Geometry: final body of the model. Coordinates: model frame, mm. Give positions to 0.01 mm unless a question says otherwise; leave off trailing zeros. Answer in a Markdown table with one row per item. Add a question column.
Autodesk Inventor part; units mm, degrees
ref_plane "C1_XY" through (0, 0, 0) normal (0, 0, 1) x (1, 0, 0)
ref_plane "C1_YZ" through (0, 0, 0) normal (1, 0, 0) x (0, 1, 0)
ref_plane "C1_ZX" through (0, 0, 0) normal (0, 1, 0) x (0, 0, 1)
sketch "Sketch_1" plane through (0, 0, 0) normal (0, 0, 1) x (1, 0, 0)
  line L0 (-15, 4) -> (-13, 4)
  line L1 (-13, 4) -> (-13, 8.25)
  line L2 (-13, 8.25) -> (-9.6642, 8.25)
  line L3 (-9.6642, 8.25) -> (-6, 4.5858)
  line L4 (-6, 4.5858) -> (-6, 0.5196)
  line L5 (-6, 0.5196) -> (-5.7, 0)
  line L6 (-5.7, 0) -> (-6, -0.5196)
  line L7 (-6, -0.5196) -> (-6, -4.5858)
  line L8 (-6, -4.5858) -> (-9.6642, -8.25)
  line L9 (-9.6642, -8.25) -> (-13, -8.25)
  line L10 (-13, -8.25) -> (-13, -4)
  line L11 (-13, -4) -> (-15, -4)
  line L12 (-15, -4) -> (-15, -13)
  arc A0 (-15, -13) -> (-13, -15) centre (-13, -13) ccw
  line L13 (-13, -15) -> (-4, -15)
  line L14 (-4, -15) -> (-4, -13)
  line L15 (-4, -13) -> (-8.25, -13)
  line L16 (-8.25, -13) -> (-8.25, -9.6642)
  line L17 (-8.25, -9.6642) -> (-4.5858, -6)
  line L18 (-4.5858, -6) -> (-0.5196, -6)
  line L19 (-0.5196, -6) -> (0, -5.7)
  line L20 (0, -5.7) -> (0.5196, -6)
  line L21 (0.5196, -6) -> (4.5858, -6)
  line L22 (4.5858, -6) -> (8.25, -9.6642)
  line L23 (8.25, -9.6642) -> (8.25, -13)
  line L24 (8.25, -13) -> (4, -13)
  line L25 (4, -13) -> (4, -15)
  line L26 (4, -15) -> (13, -15)
  arc A1 (13, -15) -> (15, -13) centre (13, -13) ccw
  line L27 (15, -13) -> (15, -4)
  line L28 (15, -4) -> (13, -4)
  line L29 (13, -4) -> (13, -8.25)
  line L30 (13, -8.25) -> (9.6642, -8.25)
  line L31 (9.6642, -8.25) -> (6, -4.5858)
  line L32 (6, -4.5858) -> (6, -0.5196)
  line L33 (6, -0.5196) -> (5.7, 0)
  line L34 (5.7, 0) -> (6, 0.5196)
  line L35 (6, 0.5196) -> (6, 4.5858)
  line L36 (6, 4.5858) -> (9.6642, 8.25)
  line L37 (9.6642, 8.25) -> (13, 8.25)
  line L38 (13, 8.25) -> (13, 4)
  line L39 (13, 4) -> (15, 4)
  line L40 (15, 4) -> (15, 13)
  arc A2 (15, 13) -> (13, 15) centre (13, 13) ccw
  line L41 (13, 15) -> (4, 15)
  line L42 (4, 15) -> (4, 13)
  line L43 (4, 13) -> (8.25, 13)
  line L44 (8.25, 13) -> (8.25, 9.6642)
  line L45 (8.25, 9.6642) -> (4.5858, 6)
  line L46 (4.5858, 6) -> (0.5196, 6)
  line L47 (0.5196, 6) -> (0, 5.7)
  line L48 (0, 5.7) -> (-0.5196, 6)
  line L49 (-0.5196, 6) -> (-4.5858, 6)
  line L50 (-4.5858, 6) -> (-8.25, 9.6642)
  line L51 (-8.25, 9.6642) -> (-8.25, 13)
  line L52 (-8.25, 13) -> (-4, 13)
  line L53 (-4, 13) -> (-4, 15)
  line L54 (-4, 15) -> (-13, 15)
  arc A3 (-13, 15) -> (-15, 13) centre (-13, 13) ccw
  line L55 (-15, 13) -> (-15, 4)
extrude "Extrusion1" add sketch "Sketch_1" against normal blind 750
sketch "Sketch2" plane through (0, 0, -750) normal (0, 0, -1) x (-1, 0, 0)
  point P0 (0, 0)
hole "Hole1" at (0, 0, -750) direction (0, 0, 1) diameter 6.8 depth 750
sketch "Sketch3" plane through (0, 0, -750) normal (0, 0, -1) x (-1, 0, 0)
  point P0 (-11.6, 11.6)
hole "Hole2" at (11.6, 11.6, -750) direction (0, 0, 1) diameter 4.2 depth 750
pattern_linear "Rectangular Pattern1" count 2 spacing 23.2 along (-1, 0, 0) count 2 spacing 23.2 along (0, -1, 0) of "Hole2"
ref_plane "C1_XY" through (0, 0, 0) normal (0, 0, 1) x (1, 0, 0)
ref_plane "C1_YZ" through (0, 0, 0) normal (1, 0, 0) x (0, 1, 0)
ref_plane "C1_ZX" through (0, 0, 0) normal (0, 1, 0) x (0, 0, 1)
ref_plane "to_frame_cap1_XY" through (0, 0, 0) normal (0, 0, 1) x (1, 0, 0)
ref_plane "to_frame_cap1_YZ" through (0, 0, 0) normal (1, 0, 0) x (0, 1, 0)
ref_plane "to_frame_cap1_ZX" through (0, 0, 0) normal (0, 1, 0) x (0, 0, 1)
ref_plane "to_frame_cap2_XY" through (0, 0, -750) normal (0, 0, -1) x (1, 0, 0)
ref_plane "to_frame_cap2_YZ" through (0, 0, -750) normal (1, 0, 0) x (0, -1, 0)
ref_plane "to_frame_cap2_ZX" through (0, 0, -750) normal (0, -1, 0) x (0, 0, -1)
properties part number "HFS6-3030-750"
(1) Cut plane A-A on z = -586. State how many separate pieces and enclosed holes the cut face has, then the cut area to 3 significant figures.
(2) Pin query (flat end, axial travel): pin 1 Ø4.5 at (x, z) = (1.5, -225) entering from +Y; pin 2 Ø1.2 at (x, z) = (2, -338) entering from -Y; pin 3 Ø1.2 at (y, z) = (-2.5, -304) entering from +X; pin 4 Ø2.5 at (x, y) = (-11.6, -11.6) entering from -Z. Return the tip coordinate at first contact, or that it passes through.
(3) Material intervals for line 1 along Y through (x, z) = (-12.25, -177); line 2 along X through (y, z) = (-11.6, -326.5), sorted ascending. Write a range as from..to.
Answer list:
| question | item | result |
|---|---|---|
| 1 | separate pieces | 1 |
| 1 | enclosed holes | 5 |
| 1 | area | 332 mm² |
| 2 | pin 1 | stops at y = 6 |
| 2 | pin 2 | stops at y = -6 |
| 2 | pin 3 | stops at x = 6 |
| 2 | pin 4 | passes through |
| 3 | line 1 | y = -15..-13.6, -9.6..-8.25, 8.25..9.6, 13.6..15 |
| 3 | line 2 | x = -15..-13.7, -9.5..-8.25, 8.25..9.5, 13.7..15 |
